```python
from build123d import *

# Parameters (mm, degrees)
SKETCH4_W                = 12.46
SKETCH4_H                = 17.25
BOSS_EXTRUDE3_DEPTH      = 6
SKETCH8_R                = 12.546781182
SKETCH8_R_2              = 11.15
BOSS_EXTRUDE6_DEPTH      = 8.3
BOSS_EXTRUDE6_DEPTH_BACK = 17.25
BOSS_EXTRUDE4_DEPTH      = 17.25
SKETCH6_R                = 0.75
CUT_EXTRUDE1_DEPTH       = 5
CHAMFER1_SIZE            = 0.5
CHAMFER1_SIZE2           = 0.866025404
SKETCH10_W               = 12.46
SKETCH10_H               = 23.7
CUT_EXTRUDE3_DEPTH       = 17.25
BOSS_EXTRUDE7_DEPTH      = 8.3
BOSS_EXTRUDE9_DEPTH      = 10
SKETCH20_R               = 11.15
SKETCH20_R_2             = 7.15
BOSS_EXTRUDE11_DEPTH     = 8.3
SKETCH21_R               = 10.15
SKETCH21_R_2             = 7.15
CUT_EXTRUDE7_DEPTH       = 1.3
SKETCH11_W               = 10
SKETCH11_H               = 2
CUT_EXTRUDE4_DEPTH       = 23.7
CUT_EXTRUDE8_REACH       = 37.55
SKETCH24_W               = 12.46
SKETCH24_H               = 6
BOSS_EXTRUDE10_DEPTH     = 25.093562
SKETCH18_W               = 21.5
SKETCH18_H               = 12.438292938
CUT_EXTRUDE5_DEPTH       = 2
SKETCH19_R               = 3.5
CUT_EXTRUDE6_DEPTH       = 43.5
CUT_EXTRUDE6_DEPTH_BACK  = 3
FILLET1_R                = 7
SKETCH22_R               = 6.5
BOSS_EXTRUDE12_DEPTH     = 5
SKETCH23_R               = 6.075
BOSS_EXTRUDE13_DEPTH     = 5
FILLET2_R                = 1
BOSS_EXTRUDE15_DEPTH     = 2
CUT_EXTRUDE9_REACH       = 46.5
SKETCH26_R               = 0.75
CUT_EXTRUDE10_DEPTH      = 26.093562364
SKETCH28_R               = 1.65
CUT_EXTRUDE11_DEPTH      = 5.975
SKETCH29_R               = 2.25
BOSS_EXTRUDE16_DEPTH     = 5
FILLET3_R                = 1
SKETCH30_W               = 5
SKETCH30_H               = 2.5
CUT_EXTRUDE12_DEPTH      = 26.093562364


with BuildPart() as part:
    # Sketch4 → Boss-Extrude3 (new body)
    with BuildSketch(Plane.XY):
        with Locations((0, -1.35)):
            Rectangle(SKETCH4_W, SKETCH4_H)
    extrude(amount=BOSS_EXTRUDE3_DEPTH)



with BuildPart() as body_2:
    # Sketch8 → Boss-Extrude6 (new body, two sides)
    with BuildSketch(Plane(origin=(0, -9.975, 0), x_dir=(-1, 0, 0), z_dir=(0, -1, 0))) as boss_extrude6_sk:
        with Locations((0, -23.55)):
            Circle(SKETCH8_R)
        with Locations((0, -23.55)):
            Circle(SKETCH8_R_2, mode=Mode.SUBTRACT)
    extrude(amount=BOSS_EXTRUDE6_DEPTH)
    extrude(boss_extrude6_sk.sketch, amount=-BOSS_EXTRUDE6_DEPTH_BACK)


with BuildPart() as part_1:
    add(part.part)

    add(body_2.part)  # Boss-Extrude4 merges body 2
    # Sketch5 → Boss-Extrude4 (add)
    with BuildSketch(Plane(origin=(0, 7.275, 0), x_dir=(1, 0, 0), z_dir=(0, 1, 0))):
        with BuildLine():
            Line((12.546781182, -23.55), (12.546781182, 0))
            Line((12.546781182, 0), (6.23, 0))
            Line((6.23, 0), (6.23, -29.7))
            Line((6.23, -29.7), (-6.23, -29.7))
            Line((-6.23, -29.7), (-6.23, 0))
            Line((-6.23, 0), (-12.546781182, 0))
            Line((-12.546781182, 0), (-12.546781182, -23.55))
            ThreePointArc((-12.546781182, -23.55), (0, -36.096781182), (12.546781182, -23.55))
        make_face()
    extrude(amount=-BOSS_EXTRUDE4_DEPTH)

    # Sketch6 → Cut-Extrude1 (cut)
    with BuildSketch(Plane(origin=(0, 7.275, 0), x_dir=(1, 0, 0), z_dir=(0, 1, 0))):
        with Locations((0, -3.6)):
            Circle(SKETCH6_R)
        with Locations((0, -32.1)):
            Circle(SKETCH6_R)
    extrude(amount=-CUT_EXTRUDE1_DEPTH, mode=Mode.SUBTRACT)

    # Chamfer1
    chamfer1_edges = [part_1.edges().sort_by_distance(p)[0] for p in [
        (-0.75, 7.275, 3.6),
        (-0.75, 7.275, 32.1),
    ]]
    chamfer1_side = [part_1.faces().sort_by_distance(p)[0] for p in [
        (0, 7.275, 35.657160381),
    ]]
    chamfer(chamfer1_edges, length=CHAMFER1_SIZE, length2=CHAMFER1_SIZE2, reference=chamfer1_side[0])

    # Sketch10 → Cut-Extrude3 (cut)
    with BuildSketch(Plane(origin=(0, 7.275, 0), x_dir=(1, 0, 0), z_dir=(0, 1, 0))):
        with Locations((0, -17.85)):
            Rectangle(SKETCH10_W, SKETCH10_H)
    extrude(amount=-CUT_EXTRUDE3_DEPTH, mode=Mode.SUBTRACT)

    # Sketch13 → Boss-Extrude7 (add)
    with BuildSketch(Plane.XZ.offset(18.275)):
        with BuildLine():
            Line((-12.546781182, 23.55), (-12.546781182, 0))
            Line((-12.546781182, 0), (12.546781182, 0))
            Line((12.546781182, 0), (12.546781182, 23.55))
            ThreePointArc((12.546781182, 23.55), (0, 11.003218818), (-12.546781182, 23.55))
        make_face()
    extrude(amount=-BOSS_EXTRUDE7_DEPTH)

    # Sketch15 → Boss-Extrude9 (add)
    with BuildSketch(Plane(origin=(0, 7.275, 0), x_dir=(1, 0, 0), z_dir=(0, 1, 0))):
        with BuildLine():
            Line((-12.546781182, 0), (12.546781182, 0))
            Line((12.546781182, 0), (12.546781182, -23.55))
            ThreePointArc((12.546781182, -23.55), (0, -36.096781182), (-12.546781182, -23.55))
            Line((-12.546781182, -23.55), (-12.546781182, 0))
        make_face()
        with BuildLine():
            Line((-6.23, -0.8), (6.23, -0.8))
            Line((6.23, -0.8), (6.23, -33))
            ThreePointArc((6.23, -33), (5.790660172, -34.060660172), (4.73, -34.5))
            Line((4.73, -34.5), (-4.73, -34.5))
            ThreePointArc((-4.73, -34.5), (-5.790660172, -34.060660172), (-6.23, -33))
            Line((-6.23, -33), (-6.23, -0.8))
        make_face(mode=Mode.SUBTRACT)
    extrude(amount=BOSS_EXTRUDE9_DEPTH)

    # Sketch20 → Boss-Extrude11 (add)
    with BuildSketch(Plane.XZ.offset(18.275)):
        with Locations((0, 23.55)):
            Circle(SKETCH20_R)
        with Locations((0, 23.55)):
            Circle(SKETCH20_R_2, mode=Mode.SUBTRACT)
    extrude(amount=-BOSS_EXTRUDE11_DEPTH)

    # Sketch21 → Cut-Extrude7 (cut)
    with BuildSketch(Plane.XZ.offset(18.275)):
        with Locations((0, 23.55)):
            Circle(SKETCH21_R)
        with Locations((0, 23.55)):
            Circle(SKETCH21_R_2, mode=Mode.SUBTRACT)
    extrude(amount=-CUT_EXTRUDE7_DEPTH, mode=Mode.SUBTRACT)

    # Sketch11 → Cut-Extrude4 (cut)
    with BuildSketch(Plane.XY.offset(29.7)):
        with Locations((0, -10.975)):
            Rectangle(SKETCH11_W, SKETCH11_H)
    extrude(amount=-CUT_EXTRUDE4_DEPTH, mode=Mode.SUBTRACT)

    # Sketch24 → Cut-Extrude8 (cut, up to next)
    with BuildSketch(Plane.XZ.offset(18.275), mode=Mode.PRIVATE) as cut_extrude8_sk1:
        with Locations((0, 9)):
            Rectangle(SKETCH24_W, SKETCH24_H)
    cut_extrude8_tool1 = extrude(cut_extrude8_sk1.sketch, amount=-CUT_EXTRUDE8_REACH, mode=Mode.PRIVATE) & part_1.part
    add(cut_extrude8_tool1.solids().sort_by_distance((0, -18.275, 9))[0], mode=Mode.SUBTRACT)

    # Sketch17 → Boss-Extrude10 (add)
    with BuildSketch(Plane(origin=(-12.546781182, 4.728218818, 0), x_dir=(0, -1, 0), z_dir=(1, 0, 0))):
        Polygon((26.978218818, 26.5), (26.978218818, 0), (-17.521781182, 0), (-17.521781182, 26.5), (-13.521781182, 26.5), (-13.521781182, 5), (22.978218818, 5), (22.978218818, 26.5), align=None)
    extrude(amount=BOSS_EXTRUDE10_DEPTH)

    # Sketch18 → Cut-Extrude5 (cut)
    with BuildSketch(Plane.ZX.offset(-18.25)):
        with Locations((-15.75, 0)):
            Rectangle(SKETCH18_W, SKETCH18_H)
    extrude(amount=-CUT_EXTRUDE5_DEPTH, mode=Mode.SUBTRACT)

    # Sketch19 → Cut-Extrude6 (cut, two sides)
    with BuildSketch(Plane.ZX.offset(-20.25)) as cut_extrude6_sk:
        with Locations((-20, 0)):
            Circle(SKETCH19_R)
    extrude(amount=CUT_EXTRUDE6_DEPTH, mode=Mode.SUBTRACT)
    extrude(cut_extrude6_sk.sketch, amount=-CUT_EXTRUDE6_DEPTH_BACK, mode=Mode.SUBTRACT)

    # Fillet1
    fillet1_edges = [part_1.edges().sort_by_distance(p)[0] for p in [
        (12.546780818, -20.25, -26.5),
        (-12.546781182, -20.25, -26.5),
        (-12.546781182, 20.25, -26.5),
        (12.546780818, 20.25, -26.5),
    ]]
    fillet(fillet1_edges, radius=FILLET1_R)

    # Sketch22 → Boss-Extrude12 (add)
    with BuildSketch(Plane(origin=(0, 22.25, 0), x_dir=(1, 0, 0), z_dir=(0, 1, 0))):
        with Locations((0, 20)):
            Circle(SKETCH22_R)
    extrude(amount=-BOSS_EXTRUDE12_DEPTH)

    # Sketch23 → Boss-Extrude13 (add)
    with BuildSketch(Plane.XZ.offset(-17.25)):
        with Locations((0, -20)):
            Circle(SKETCH23_R)
    extrude(amount=BOSS_EXTRUDE13_DEPTH)

    # Fillet2
    fillet2_edges = [part_1.edges().sort_by_distance(p)[0] for p in [
        (-6.075, 12.25, -20),
    ]]
    fillet(fillet2_edges, radius=FILLET2_R)

    # Sketch25 → Boss-Extrude15 (add)
    with BuildSketch(Plane(origin=(0, -20.25, 0), x_dir=(1, 0, 0), z_dir=(0, 1, 0))):
        Polygon((-6.219146469, 5), (-2.5, 5), (-3.1585, 20), (-3.44385, 26.5), (-6.219146469, 26.5), align=None)
        Polygon((6.219146469, 5), (2.5, 5), (3.1585, 20), (3.44385, 26.5), (6.219146469, 26.5), align=None)
    extrude(amount=BOSS_EXTRUDE15_DEPTH)

    # Sketch26 → Cut-Extrude9 (cut, up to next)
    with BuildSketch(Plane(origin=(0, -22.25, 0), x_dir=(-1, 0, 0), z_dir=(0, -1, 0)), mode=Mode.PRIVATE) as cut_extrude9_sk1:
        with Locations((0, 10)):
            Circle(SKETCH26_R)
    cut_extrude9_tool1 = extrude(cut_extrude9_sk1.sketch, amount=-CUT_EXTRUDE9_REACH, mode=Mode.PRIVATE) & part_1.part
    add(cut_extrude9_tool1.solids().sort_by_distance((0, -22.25, -10))[0], mode=Mode.SUBTRACT)

    # Sketch27 → Cut-Extrude10 (cut, through all)
    with BuildSketch(Plane.ZY.offset(12.546781182)):
        Polygon((36.096781182, 17.275), (-10.020668602, 17.275), (-10.020668602, 5.331631915), (-33.329469664, 5.331631915), (-33.329469664, -27.204993615), (36.096781182, -27.204993615), align=None)
    extrude(amount=-CUT_EXTRUDE10_DEPTH, mode=Mode.SUBTRACT)

    # Sketch28 → Cut-Extrude11 (cut, through all)
    with BuildSketch(Plane.XZ.offset(-17.275)):
        with Locations((-8, -2.5)):
            Circle(SKETCH28_R)
        with Locations((8, -2.5)):
            Circle(SKETCH28_R)
    extrude(amount=-CUT_EXTRUDE11_DEPTH, mode=Mode.SUBTRACT)

    # Sketch29 → Boss-Extrude16 (add)
    with BuildSketch(Plane.XZ.offset(-17.275)):
        with Locations((0, -2.5)):
            Circle(SKETCH29_R)
    extrude(amount=BOSS_EXTRUDE16_DEPTH)

    # Fillet3
    fillet3_edges = [part_1.edges().sort_by_distance(p)[0] for p in [
        (-2.25, 12.275, -2.5),
    ]]
    fillet(fillet3_edges, radius=FILLET3_R)

    # Sketch30 → Cut-Extrude12 (cut, through all)
    with BuildSketch(Plane(origin=(12.546781182, 0, 0), x_dir=(0, 0, -1), z_dir=(1, 0, 0))):
        with Locations((2.5, 21)):
            Rectangle(SKETCH30_W, SKETCH30_H)
    extrude(amount=-CUT_EXTRUDE12_DEPTH, mode=Mode.SUBTRACT)


solid = part_1.part
```
Here's how the part is built. I have some questions about the finished solid (model axes, mm). A direction names the side the tool comes from. Round coordinates to 2 decimals unless told otherwise and drop trailing zeros. Order: outer loops, then holes, each group sorted by start corner. A loop starts at its lowest first (then second) coordinate and runs counter-clockwise, first axis right, second up. Notation, with made-up numbers: M -8,52.5 L 51,52.5 A13 ccw 51,61.5 Z; hole C 20,-22 d5. An arc over 180 degrees is marked long. One line per question, with ' | ' between items.
1) I want a section at D-D, the plane x = 10.5. Write out the boundary of the cut face in (y, z) (3 decimals).
Working result:
outline: M 17.275,-5 L 18.25,-5 L 18.25,-24.446 L 22.25,-24.446 L 22.25,-5 L 19.75,-5 L 19.75,0 L 17.275,0 Z
2) I want a section at C-C, the plane y = 21.75. Write out the boundary of the cut face in (x, z).
Working result:
outline: M -12.55,-19.5 A7 ccw -5.55,-26.5 L 5.55,-26.5 A7 ccw 12.55,-19.5 L 12.55,-5 L -12.55,-5 Z
3) I need wall thicknesses on line 1 along Z through (x, y) = (8, 17.9); line 2 along Y through (x, z) = (11.25, -22.25); line 3 along Z through (x, y) = (1.5, 20.25). Which ranges of each line are inside material? Lowest first, please.
Working result:
line 1: -5 to -4.15, -0.85 to 0 | line 2: 18.25 to 22.25 | line 3: -26.5 to -5
4) If we mould it in two halves opening along X, with no side actions, what happens to faces 4 (the face through (6.784, 18.495, -1.385)), 5 (the face through (0, 12.25, -20)), 6 (the face through (-10.551, 20.222, -24.395))? For each: +X half, -X half, draft (parallel to the pull), parting line (faces both ways), or undercut.
Working result:
face 4: undercut | face 5: draft | face 6: -X half
5) I want a section at B-B, the plane x = -8. Write out the boundary of the cut face in (y, z) (3 decimals), then the cut area to 3 significant figures.
Working result:
outline: M 17.275,-5 L 18.25,-5 L 18.25,-26.056 L 22.25,-26.056 L 22.25,-5 L 19.75,-5 L 19.75,-4.15 L 17.275,-4.15 Z; M 17.275,-0.85 L 19.75,-0.85 L 19.75,0 L 17.275,0 Z | area: 88.4 mm²
6) I want a section at A-A, the plane z = -2.5. Write out the boundary of the cut face in (x, y) (3 decimals), then the cut area to 3 significant figures.
Working result:
outline: M -12.547,17.275 L -9.65,17.275 L -9.65,19.75 L -12.547,19.75 Z; M -6.35,17.275 L -2.25,17.275 L -2.25,13.275 A1 ccw -1.25,12.275 L 1.25,12.275 A1 ccw 2.25,13.275 L 2.25,17.275 L 6.35,17.275 L 6.35,19.75 L -6.35,19.75 Z; M 9.65,17.275 L 12.547,17.275 L 12.547,19.75 L 9.65,19.75 Z | area: 67.8 mm²
7) For pin 1 Ø2 at (x, z) = (8, -2.5) entering from -Y; pin 2 Ø5 at (x, z) = (-0.5, -7) entering from -Y; pin 3 Ø0.8 at (x, z) = (0, -2) entering from -Y (3 decimals); pin 4 Ø1.5 at (x, z) = (5.5, -3) entering from +Y, each with a flat end and sliding along its axis, tell me the tip position at first contact or that it passes through.
Working result:
pin 1: through | pin 2: y = 12.65 | pin 3: y = 12.275 | pin 4: y = 19.75
8) For faces 1 (the face through (0, 19.75, -2)), 2 (the face through (0, 18, -5)), 3 (the face through (-1.32, 15.28, -25.93)), which set-ups out of +Z, -Z, +X, -X, +Y, -Y let a thin tool reach every point of the face, with its end or its side?
Working result:
face 1: +Z, +X, -X, +Y | face 2: +X, -X, -Y | face 3: -Y
